from build123d import *

# Parameters (mm, degrees)
SKETCH_1_R                   = 25
SKETCH_1_R_2                 = 17.5
EXTRUDE_1_DEPTH              = 15
HOLE_WIZARD_M102_D           = 8.5
HOLE_WIZARD_M102_DEPTH       = 24.946342369
HOLE_WIZARD_M102_CSINK_D     = 10.05
HOLE_WIZARD_M102_CSINK_ANGLE = 90
HOLE_WIZARD_M102_TIP         = 2.553657631


with BuildPart() as part:
    # Эскиз1 → Бобышка-Вытянуть1 (new body)
    with BuildSketch(Plane.XY):
        Circle(SKETCH_1_R)
        Circle(SKETCH_1_R_2, mode=Mode.SUBTRACT)
    extrude(amount=EXTRUDE_1_DEPTH)

    # Отверстие обработанное метчиком M102
    with Locations(Plane(origin=(1.106433423, 17.464987978, 7.5), x_dir=(-0.997999313042, 0.063224767047, 0), z_dir=(-0.063224767047, -0.997999313042, 0))):
        with Locations((0, 0)):
            CounterSinkHole(HOLE_WIZARD_M102_D / 2, HOLE_WIZARD_M102_CSINK_D / 2, depth=HOLE_WIZARD_M102_DEPTH, counter_sink_angle=HOLE_WIZARD_M102_CSINK_ANGLE)
            with Locations((0, 0, -(HOLE_WIZARD_M102_DEPTH + HOLE_WIZARD_M102_TIP / 2))):  # 118° drill point
                Cone(0, HOLE_WIZARD_M102_D / 2, HOLE_WIZARD_M102_TIP, mode=Mode.SUBTRACT)


solid = part.part
For this review, take the finished solid that the model builds, in its own axes (mm). A direction names the side the tool comes from. Round coordinates to 2 decimals unless told otherwise and drop trailing zeros. Loops run counter-clockwise (first coordinate to the right, second up) from the corner with the lowest first, then second, coordinate; pieces in that order, holes last. Notation, with made-up numbers: (49.5, 27) - (103.5, 27) arc R14 ccw to (103.5, 42) - close; hole circle Ø3 at (-37.5, -19). An arc over 180 degrees is marked (long way). One line per question, with ' | ' between items.
Q1. Take a section at A-A (y = 0). Give the boundary of the cut face in (x, z), and give its area (3 significant figures).
Taken from the geometry:
outline: (-25, 0) - (-17.5, 0) - (-17.5, 15) - (-25, 15) - close; (17.5, 0) - (25, 0) - (25, 15) - (17.5, 15) - close | area: 225 mm²
Q2. Take a section at D-D (x = 0). State how many separate pieces and enclosed holes the cut face has, and give its area (3 significant figures).
Taken from the geometry:
separate pieces: 3 | enclosed holes: 0 | area: 164 mm²
Q3. Take a section at C-C (x = -6.5). Give the boundary of the cut face in (y, z).
Taken from the geometry:
outline: (-24.14, 0) - (-16.25, 0) - (-16.25, 15) - (-24.14, 15) - close; (16.25, 0) - (24.14, 0) - (24.14, 15) - (16.25, 15) - close
Q4. The part is to be moulded in two halves that separate along Y. For faces 3 (the flat face through (-17, -5, 0)), 4 (the cylindrical face through (23.846, 7.509, 7.395)), 5 (the cylindrical face through (-3.794, -17.084, 7.395)), say which applies: released by +Y, released by -Y, zero draft, split by the parting line, or undercut.
Taken from the geometry:
face 3: zero draft | face 4: split by the parting line | face 5: undercut
Q5. For line 1 along Y through (x, z) = (0, 6.25); line 2 along Y through (x, z) = (-2.5, 13.25); line 3 along X through (y, z) = (-1, 11.25), list the stretches that pass through material, from the lowest coordinate up. Write a range as [from, to].
Taken from the geometry:
line 1: y = [-25, -17.5] | line 2: y = [-24.87, -17.32], [17.32, 24.87] | line 3: x = [-24.98, -17.47], [17.47, 24.98]
Q6. Tool access review of faces 1 (the cylindrical face through (-3.926, 17.491, 7.61)), 2 (the flat face through (-17, -5, 15)): name each direction out of +Z, -Z, +X, -X, +Y, -Y from which nothing blocks a thin tool from reaching the whole face with its end or side.
Taken from the geometry:
face 1: none | face 2: +Z, +X, -X, +Y, -Y
Q7. Take a section at B-B (z = 14). Give the boundary of the cut face in (x, y).
Taken from the geometry:
outline: circle Ø50 at (0, 0); hole circle Ø35 at (0, 0)
Q8. For pin 1 (1 mm diameter, centred on y = -12, z = 11, fed in from +X); pin 2 (8 mm diameter, centred on x = 9.5, z = 6.5, fed in from -Y); pin 3 (1 mm diameter, centred on x = 13, z = 9.5, fed in from -Y), all flat-tipped, find the tip position at first contact; note any pin that passes through.
Taken from the geometry:
pin 1: stops at x = 22.2 | pin 2: stops at y = -24.39 | pin 3: stops at y = -21.65
